Verification items for the finished model (mm, model axes). A direction names the side the tool comes from. Round coordinates to 2 decimals unless told otherwise and drop trailing zeros. Loops run counter-clockwise (first coordinate to the right, second up) from the corner with the lowest first, then second, coordinate; pieces in that order, holes last. Notation, with made-up numbers: M 73.5,-33.75 L 121.5,-33.75 A26 ccw 121.5,-11.75 Z; hole C 65,8 d5. An arc over 180 degrees is marked long. One line per item, written item: value.
from build123d import *

# Parameters (mm, degrees)
F0_W         = 52
F0_H         = 60
F1_DEPTH     = 5
F2_R         = 10
F3_R         = 2.25
F4_DEPTH     = 25
F6_DEPTH     = 2
F7_W         = 24
F7_H         = 25
F8_DEPTH     = 25
F10_DEPTH    = 40.501
F11_R        = 5.25
F12_DEPTH    = 25.3474527662
F13_R        = 10
F13_R_2      = 5.25
F14_DEPTH    = 3
F16_R        = 10
F17_DEPTH    = 12
F18_DEPTH    = 25.001
F19_F1_R     = 5
F19_T2_DEPTH = 31.5358983849
F19_T4_DEPTH = 28.6534286629
F19_T6_DEPTH = 42.117530278
F19_T8_DEPTH = 49


# Not quite as in the source:
# - a fillet or chamfer that OpenCascade refuses, or shapes differently, is made with other operations: its cross-section is extruded or revolved along the edge and cut away or added


with BuildPart() as f1:
    # F0 (on Top) → F1 (new body)
    with BuildSketch(Plane.XY):
        Rectangle(F0_W, F0_H)
    extrude(amount=F1_DEPTH)

    # F2
    f2_edges = [f1.edges().sort_by_distance(p)[0] for p in [
        (26, -30, 2.5),
        (-26, -30, 2.5),
        (26, 30, 2.5),
        (-26, 30, 2.5),
    ]]
    fillet(f2_edges, radius=F2_R)

    # F3 (on face) → F4 (cut)
    with BuildSketch(Plane.XY.offset(5)):
        with Locations((-16, -20)):
            Circle(F3_R)
        with Locations((16, -20)):
            Circle(F3_R)
        with Locations((-16, 20)):
            Circle(F3_R)
        with Locations((16, 20)):
            Circle(F3_R)
    extrude(amount=-F4_DEPTH, mode=Mode.SUBTRACT)

    # F5 (on face) → F6 (cut)
    with BuildSketch(Plane.XY.offset(5)):
        Polygon((-16, -15.6698729811), (-19.75, -17.8349364905), (-19.75, -22.1650635095), (-16, -24.3301270189), (-12.25, -22.1650635095), (-12.25, -17.8349364905), align=None)
        Polygon((-12.25, 22.1650635095), (-16, 24.3301270189), (-19.75, 22.1650635095), (-19.75, 17.8349364905), (-16, 15.6698729811), (-12.25, 17.8349364905), align=None)
        Polygon((19.75, -17.8349364905), (16, -15.6698729811), (12.25, -17.8349364905), (12.25, -22.1650635095), (16, -24.3301270189), (19.75, -22.1650635095), align=None)
        Polygon((19.75, 22.1650635095), (16, 24.3301270189), (12.25, 22.1650635095), (12.25, 17.8349364905), (16, 15.6698729811), (19.75, 17.8349364905), align=None)
    extrude(amount=-F6_DEPTH, mode=Mode.SUBTRACT)

    # F7 (on face) → F8 (join)
    with BuildSketch(Plane.XY.offset(5)):
        with Locations((-2.5, 17.5)):
            Rectangle(F7_W, F7_H)
    extrude(amount=F8_DEPTH)

    # F9 (on face) → F10 (cut, through all)
    with BuildSketch(Plane(origin=(-14.5, 0, 0), x_dir=(0, -1, 0), z_dir=(-1, 0, 0))):
        Polygon((-12.882469722, 30), (-5, 5), (-5, 30), align=None)
    extrude(amount=-F10_DEPTH, mode=Mode.SUBTRACT)

    # F11 (on face) → F12 (cut, through all)
    with BuildSketch(Plane(origin=(0, 3.1139390198, -0.9818212016), x_dir=(1, 0, 0), z_dir=(0, -0.9537169507, 0.3007057995))):
        with Locations((-2.5, 19.3787278155)):
            Circle(F11_R)
    extrude(amount=-F12_DEPTH, mode=Mode.SUBTRACT)

    # F13 (on face) → F14 (cut)
    with BuildSketch(Plane(origin=(0, 3.1139390198, -0.9818212016), x_dir=(1, 0, 0), z_dir=(0, -0.9537169507, 0.3007057995))):
        with Locations((-2.5, 19.3787278155)):
            Circle(F13_R)
        with Locations((-2.5, 19.3787278155)):
            Circle(F13_R_2, mode=Mode.SUBTRACT)
    extrude(amount=-F14_DEPTH, mode=Mode.SUBTRACT)

    # F16 (on offset) → F17 (cut)
    with BuildSketch(Plane(origin=(0, 29.8180136408, -9.4015835877), x_dir=(1, 0, 0), z_dir=(0, -0.9537169507, 0.3007057995))):
        with Locations((-2.5, 19.3787278155)):
            Circle(F16_R)
    extrude(amount=F17_DEPTH, mode=Mode.SUBTRACT)

    # F5 (on face) → F18 (cut, through all)
    with BuildSketch(Plane.XY.offset(5)):
        Polygon((-16, -15.6698729811), (-19.75, -17.8349364905), (-19.75, -22.1650635095), (-16, -24.3301270189), (-12.25, -22.1650635095), (-12.25, -17.8349364905), align=None)
        Polygon((-12.25, 22.1650635095), (-16, 24.3301270189), (-19.75, 22.1650635095), (-19.75, 17.8349364905), (-16, 15.6698729811), (-12.25, 17.8349364905), align=None)
        Polygon((19.75, -17.8349364905), (16, -15.6698729811), (12.25, -17.8349364905), (12.25, -22.1650635095), (16, -24.3301270189), (19.75, -22.1650635095), align=None)
        Polygon((19.75, 22.1650635095), (16, 24.3301270189), (12.25, 22.1650635095), (12.25, 17.8349364905), (16, 15.6698729811), (19.75, 17.8349364905), align=None)
    extrude(amount=F18_DEPTH, mode=Mode.SUBTRACT)

    # F19: fillet of radius 5 on 5 edges, made by hand

    # F19_f1
    f19_f1_edges = [f1.edges().sort_by_distance(p)[0] for p in [
        (-2.5, 5, 5),
    ]]
    fillet(f19_f1_edges, radius=F19_F1_R)

    # F19_s3 → F19_t2 (cut)
    with BuildSketch(Plane.XZ.offset(-42.5)):
        with BuildLine():
            ThreePointArc((-14.5, 25), (-13.0355339059, 28.5355339059), (-9.5, 30))
            Line((-9.5, 30), (-9.5, 30.1))
            Line((-9.5, 30.1), (-14.6, 30.1))
            Line((-14.6, 30.1), (-14.6, 25))
            Line((-14.6, 25), (-14.5, 25))
        make_face()
    extrude(amount=F19_T2_DEPTH, mode=Mode.SUBTRACT)

    # F19_s5 → F19_t4 (cut)
    with BuildSketch(Plane.XZ.offset(-29.0358983849)):
        with BuildLine():
            ThreePointArc((-14.5, 25), (-13.0355339059, 28.5355339059), (-9.5, 30))
            Line((-9.5, 30), (-9.5, 30.1))
            Line((-9.5, 30.1), (-14.6, 30.1))
            Line((-14.6, 30.1), (-14.6, 25))
            Line((-14.6, 25), (-14.5, 25))
        make_face()
    extrude(amount=F19_T4_DEPTH, mode=Mode.SUBTRACT)

    # F19_s7 → F19_t6 (cut)
    with BuildSketch(Plane.XZ.offset(-42.5)):
        with BuildLine():
            ThreePointArc((9.5, 25), (8.0355339059, 28.5355339059), (4.5, 30))
            Line((4.5, 30), (4.5, 30.1))
            Line((4.5, 30.1), (9.6, 30.1))
            Line((9.6, 30.1), (9.6, 25))
            Line((9.6, 25), (9.5, 25))
        make_face()
    extrude(amount=F19_T6_DEPTH, mode=Mode.SUBTRACT)

    # F19_s9 → F19_t8 (cut)
    with BuildSketch(Plane.YZ.offset(-27)):
        with BuildLine():
            ThreePointArc((30, 25), (28.5355339059, 28.5355339059), (25, 30))
            Line((25, 30), (25, 30.1))
            Line((25, 30.1), (30.1, 30.1))
            Line((30.1, 30.1), (30.1, 25))
            Line((30.1, 25), (30, 25))
        make_face()
    extrude(amount=F19_T8_DEPTH, mode=Mode.SUBTRACT)


solid = f1.part
(1) Sectioned sample at A-A on x = 2. Enter the section's corners in (y, z), and give its area (3 significant figures).
Completed:
outline: M -30,0 L 30,0 L 30,1.5 L 21.52,4.17 L 23.39,10.11 L 10.99,14.02 L 9.12,8.08 L 6.26,8.98 L 6.1,8.5 A5 cw 1.33,5 L -30,5 Z; M 11.63,26.02 L 14.49,25.11 L 12.62,19.18 L 25.01,15.27 L 26.89,21.21 L 30,20.22 L 30,25 A5 ccw 25,30 L 12.88,30 Z
area: 591 mm^2
(2) Sectioned sample at B-B on y = -23. Enter the section's corners in (x, z), and give its area (3 significant figures).
Completed:
outline: M -25.54,0 L 25.54,0 L 25.54,5 L 18.3,5 L 18.3,3 L 13.7,3 L 13.7,5 L -13.7,5 L -13.7,3 L -18.3,3 L -18.3,5 L -25.54,5 Z
area: 237 mm^2
(3) Depth check by flat-ended pin: pin 1 Ø1 at (x, y) = (-19.5, -18.5) entering from +Z; pin 2 Ø8 at (x, z) = (20.5, 4) entering from +Y; pin 3 Ø6 at (y, z) = (10.5, 10.5) entering from +X. Enter the tip coordinate at first touch or a pass-through.
Completed:
pin 1: stops at z = 5
pin 2: stops at y = 29.99
pin 3: stops at x = 9.5
(4) Tool access check on faces 1 (the face through (-13.265, 22.751, 13.363)), 2 (the face through (26, 0, 2)). Record the directions out of +Z, -Z, +X, -X, +Y, -Y that give a thin tool (end or side, any length) a straight path to the whole face; none if there is none.
Completed:
face 1: +Z
face 2: +Z, -Z, +X, +Y, -Y
(5) Sectioned sample at D-D on y = -2. Enter the section's corners in (x, z), and give its area (3 significant figures).
Completed:
outline: M -26,0 L 26,0 L 26,5 L -26,5 Z
area: 260 mm^2
(6) Mould release check, pull along Z, two halves, no side actions. Record for faces 3 (the face through (1.804, 22.906, 8.583)), 4 (the face through (1.804, 10.508, 12.493)), 5 (the face through (-11.66, 20.78, 29.51)), 6 (the face through (9.5, 19, 15)): +Z half, -Z half, draft (parallel to the pull), parting line (faces both ways), or undercut.
Completed:
face 3: undercut
face 4: undercut
face 5: +Z half
face 6: draft
(7) Sectioned sample at C-C on x = -21. Enter the section's corners in (y, z).
Completed:
outline: M -28.66,0 L 28.66,0 L 28.66,5 L -28.66,5 Z
(8) Thickness scan on L1, parallel to Y at x = -16, z = 1.95; L2, parallel to Z at x = -9, y = -21; L3, parallel to Z at x = 1.5, y = 18. Record the ranges inside material, lowest first. Write a range as from..to.
Completed:
L1: y = -30..-22.25, -17.75..17.75, 22.25..30
L2: z = 0..5
L3: z = 0..11.08, 18.21..30
